Input: dimensioned drawing with shaded views. Units: mm. Origin: part minimum x, y, z. A direction names the side the tool comes from. Give positions to 0.01 mm unless a question says otherwise; leave off trailing zeros. Order: outer loops, then holes, each group sorted by start corner. A loop starts at its lowest first (then second) coordinate and runs counter-clockwise, first axis right, second up. Notation, with made-up numbers: (-38, -16.75) -> (21, -16.75) arc R4 cw to (21, -9.75) -> close; hole circle Ø10 at (23.5, -12). An arc over 180 degrees is marked (long way). One line per question, with ' | ' between items. Start each with the question number.
(1) First-contact query: pin 1 Ø5 at (y, z) = (10.5, 4) entering from -X; pin 2 Ø4 at (x, y) = (2, 22) entering from +Z; pin 3 Ø4 at (y, z) = (54.5, 5.5) entering from -X. Flat tips, straight axial feed; report the tip coordinate or a pass-through.
(2) Section B-B (y = 73.5). Return loops of the section in (x, z).
(3) Set-up query: the marked faces 1 and 2. Return all of +Z, -Z, +X, -X, +Y, -Y with unobstructed straight access to the full face (end or side cutting, diameter ignored); none if empty.
(4) Section A-A (z = 7). Return loops of the section in (x, y), then the cut area to 3 significant figures.
(5) Section C-C (y = 49). Return loops of the section in (x, z).
(6) Ray query, L1, parallel to X at y = 70, z = 7; L2, parallel to X at y = 44.5, z = 5.5; L3, parallel to Z at x = 8.5, y = 73. Return the intervals inside material, ascending.
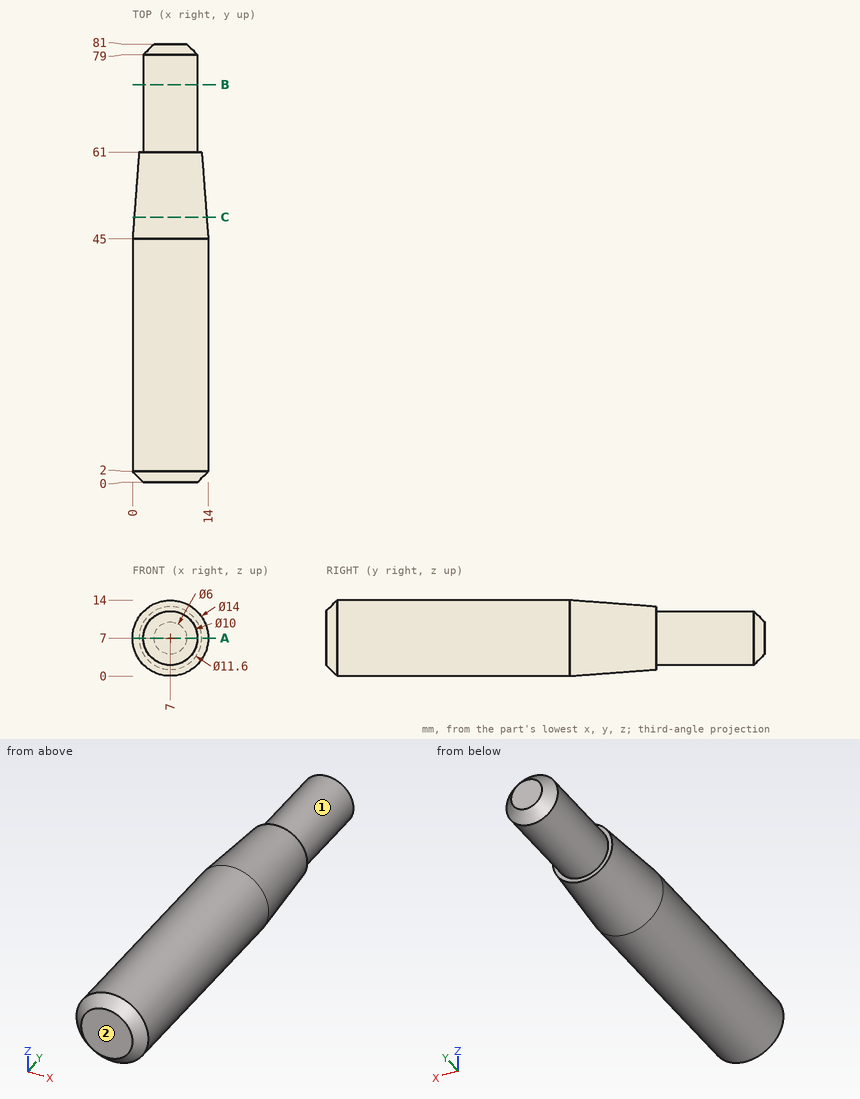
Response:
1) pin 1: stops at x = 0.02 | pin 2: stops at z = 13.32 | pin 3: stops at x = 0.6
2) outline: circle Ø10 at (7, 7)
3) face 1: +Y | face 2: +Z, -Z, +X, -X, -Y
4) outline: (0, 2) -> (2, 0) -> (12, 0) -> (14, 2) -> (14, 45) -> (12.8, 61) -> (12, 61) -> (12, 79) -> (10, 81) -> (4, 81) -> (2, 79) -> (2, 61) -> (1.2, 61) -> (0, 45) -> close | area: 1,030 mm^2
5) outline: circle Ø13.4 at (7, 7)
6) L1: x = 2 to 12 | L2: x = 0.16 to 13.84 | L3: z = 2.23 to 11.77
